Build history of the part. All positions in model axes, mm. A direction names the side the tool comes from. Give positions to 0.01 mm unless a question says otherwise; leave off trailing zeros. Order: outer loops, then holes, each group sorted by start corner. A loop starts at its lowest first (then second) coordinate and runs counter-clockwise, first axis right, second up. Notation, with made-up numbers: (59, -37) - (63, -37) arc R26 ccw to (63, -20) - close; hole circle Ø2 at (58, 53). An arc over 180 degrees is marked (long way). Use a Markdown table: item, result.
from build123d import *

# Parameters (mm, degrees)
F1_DEPTH = 42.418
F3_START = 17.526
F3_DEPTH = 7.874
F4_F1_R  = 5.08
F4_F2_R  = 5.08
F4_F3_R  = 5.08
F4_F4_R  = 5.08
F4_F5_R  = 5.08
F4_F6_R  = 5.08
F4_F7_R  = 5.08
F4_F8_R  = 5.08


# Not quite as in the source:
# - a feature of the source that left no trace in its solid (it failed there, or was rolled back) is left out


with BuildPart() as f1:
    # F0 (on Front) → F1 (new body)
    with BuildSketch(Plane.XZ):
        Polygon((5.7973779566, -73.3064366429), (29.5106887989, -30.4560707957), (4.2578388349, 11.5054417251), (-44.7083219714, 10.6165883988), (-68.4216328137, -32.2337774485), (-43.1687828497, -74.1952899693), align=None)
    extrude(amount=F1_DEPTH)

    # F2 (on Front) → F3 (join)
    with BuildSketch(Plane.XZ.offset(F3_START)):
        Polygon((-23.4186239541, 28.8229137659), (-23.4186239541, 23.4186165035), (-23.4186239541, -51.1606782675), (-20.8966191858, -54.4032603502), (-20.8966191858, 28.8229137659), align=None)
        with BuildLine():
            Line((-28.8229212165, 28.8229137659), (-23.4186239541, 28.8229137659))
            Line((-23.4186239541, 28.8229137659), (-20.8966191858, 28.8229137659))
            Line((-20.8966191858, 28.8229137659), (-15.1320351288, 28.8229137659))
            ThreePointArc((-15.1320351288, 28.8229137659), (-21.9774781726, 40.5074513695), (-28.8229212165, 28.8229137659))
        make_face()
    extrude(amount=F3_DEPTH)

    # F4: fillet of radius 5.08 on 14 edges, made by hand

    # F4_f1
    f4_f1_edges = [f1.edges().sort_by_distance(p)[0] for p in [
        (5.7973779566, -21.209, -73.3064366429),
    ]]
    fillet(f4_f1_edges, radius=F4_F1_R)

    # F4_f2
    f4_f2_edges = [f1.edges().sort_by_distance(p)[0] for p in [
        (29.5106887989, -21.209, -30.4560707957),
    ]]
    fillet(f4_f2_edges, radius=F4_F2_R)

    # F4_f3
    f4_f3_edges = [f1.edges().sort_by_distance(p)[0] for p in [
        (-43.1687828497, -21.209, -74.1952899693),
    ]]
    fillet(f4_f3_edges, radius=F4_F3_R)

    # F4_f4
    f4_f4_edges = [f1.edges().sort_by_distance(p)[0] for p in [
        (4.2578388349, -21.209, 11.5054417251),
    ]]
    fillet(f4_f4_edges, radius=F4_F4_R)

    # F4_f5
    f4_f5_edges = [f1.edges().sort_by_distance(p)[0] for p in [
        (-68.4216328137, -21.209, -32.2337774485),
    ]]
    fillet(f4_f5_edges, radius=F4_F5_R)

    # F4_f6
    f4_f6_edges = [f1.edges().sort_by_distance(p)[0] for p in [
        (-44.7083219714, -21.209, 10.6165883988),
    ]]
    fillet(f4_f6_edges, radius=F4_F6_R)

    # F4_f7
    f4_f7_edges = [f1.edges().sort_by_distance(p)[0] for p in [
        (-55.7952078317, 0, -53.2145337089),
    ]]
    fillet(f4_f7_edges, radius=F4_F7_R)

    # F4_f8
    f4_f8_edges = [f1.edges().sort_by_distance(p)[0] for p in [
        (-55.7952078317, -42.418, -53.2145337089),
    ]]
    fillet(f4_f8_edges, radius=F4_F8_R)


solid = f1.part
1) Tool access for faces 1 (the cylindrical face through (-18.41, -40.89, -72.3)), 2 (the cylindrical face through (-20.5, -1.45, 9.53)), 3 (the cylindrical face through (-20.5, -40.9, 9.6)): list every direction of +Z, -Z, +X, -X, +Y, -Y with a clear straight run to the whole face (end or side of a thin tool).
Computed:
| item | result |
|---|---|
| face 1 | -Z, +X, -Y |
| face 2 | +Z, -X, +Y |
| face 3 | +Z, -X, -Y |
2) Pin check, flat tips, straight feed: P1, Ø12, axis at x = -56.5, y = -14.5, coming from the -Z side; P2, Ø17.5, axis at x = -21.5, z = 32, coming from the +Y side; P3, Ø10, axis at x = -52.5, y = -38, coming from the +Z side. Stop position of each tip, or through.
Computed:
| item | result |
|---|---|
| P1 | stops at z = -62.01 |
| P2 | stops at y = -17.53 |
| P3 | stops at z = 5.53 |
3) Two-plate mould, pull along Z, no slides. Class faces 4 (the flat face through (-20.897, -21, 20)), 5 (the cylindrical face through (15.42, -1.45, -10)), 6 (the cylindrical face through (16.53, -40.89, -50.92)): +Z half, -Z half, draft (parallel to the pull), parting line (faces both ways), or undercut.
Computed:
| item | result |
|---|---|
| face 4 | undercut |
| face 5 | +Z half |
| face 6 | -Z half |
4) Slice it at B-B (y = -12). Write the cut outline in (x, z), and give its area (3 significant figures).
Computed:
| item | result |
|---|---|
| outline | (-67, -29.67) arc R5.08 ccw to (-66.91, -34.75) - (-44.68, -71.68) arc R5.08 ccw to (-40.24, -74.14) - (2.86, -73.36) arc R5.08 ccw to (7.22, -70.74) - (28.09, -33.02) arc R5.08 ccw to (28, -27.94) - (5.77, 8.99) arc R5.08 ccw to (1.33, 11.45) - (-41.78, 10.67) arc R5.08 ccw to (-46.13, 8.05) - close |
| area | 6,220 mm² |
5) Wall check: line 1 (X direction, y = -40.5, z = -28.5); line 2 (X direction, y = -6.5, z = -19); line 3 (Y direction, x = -7, z = -69). Give the ranges that are in metal, low to high. Write a range as from..to.
Computed:
| item | result |
|---|---|
| line 1 | x = -65.09..27.04 |
| line 2 | x = -61.1..22.62 |
| line 3 | y = -42.39..-0.03 |
6) Slice it at A-A (y = -22). Write the cut outline in (x, z), and give its area (3 significant figures).
Computed:
| item | result |
|---|---|
| outline | (-67, -29.67) arc R5.08 ccw to (-66.91, -34.75) - (-44.68, -71.68) arc R5.08 ccw to (-40.24, -74.14) - (2.86, -73.36) arc R5.08 ccw to (7.22, -70.74) - (28.09, -33.02) arc R5.08 ccw to (28, -27.94) - (5.77, 8.99) arc R5.08 ccw to (1.33, 11.45) - (-20.9, 11.05) - (-20.9, 28.82) - (-15.13, 28.82) arc R7.85 ccw (long way) to (-28.82, 28.82) - (-23.42, 28.82) - (-23.42, 11) - (-41.78, 10.67) arc R5.08 ccw to (-46.13, 8.05) - close |
| area | 6,420 mm² |
